Read the model definition and answer for the solid it produces. Units are mm, in the model's axes. Face numbers are marked on the shaded views. Coordinates: 2 decimals unless noted, no trailing zeros. Answer as a JSON object with one key per item and string values. Group by question number.
1) Given pin 1 (1.5 mm diameter, centred on y = -9.5, z = 4, fed in from +X), flat-ended and moving along its own axis, determine where the tip first touches the part or whether it passes through.
2) Consider L1, parallel to X at y = -1.25, z = 0.75; L2, parallel to Y at x = -61, z = 4.75; L3, parallel to X at y = 9.75, z = 5.25. Determine where each line is inside the solid, lowest interval first.
3) Determine the mould class of the marked faces 1, 2 and 3 for opening direction X: released by +X, released by -X, zero draft, split by the parting line, or undercut.
4) Section A-A on z = 3 is taken. Count the separate pieces of the cut face and the enclosed holes in it, and give its area (3 significant figures).
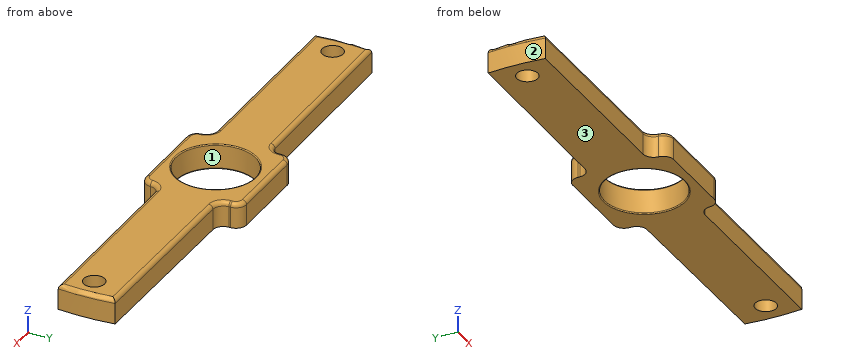
from build123d import *

# Parameters (mm, degrees)
ESQUISSE1_W             = 200
ESQUISSE1_H             = 24
BOSS_EXTRU_1_DEPTH      = 6
ESQUISSE3_R             = 9.5
ENL_V_MAT_EXTRU_1_DEPTH = 6
ESQUISSE4_R             = 114.275088212
ESQUISSE4_R_2           = 60
ENL_V_MAT_EXTRU_2_DEPTH = 6
ESQUISSE5_W             = 52.011744551
ESQUISSE5_H             = 15.54113196
ESQUISSE5_W_2           = 52.011744552
ENL_V_MAT_EXTRU_3_DEPTH = 6
CONG_1_R                = 2.5
CONG_2_R                = 2.5
CONG_3_R                = 1
CONG_4_R                = 0.25
CONG_5_R                = 0.25
ESQUISSE6_R             = 2.5
ENL_V_MAT_EXTRU_4_DEPTH = 68.365782888


with BuildPart() as part:
    # Esquisse1 → Boss.-Extru.1 (new body)
    with BuildSketch(Plane.XY):
        with Locations((-5.765391807, 0)):
            Rectangle(ESQUISSE1_W, ESQUISSE1_H)
    extrude(amount=BOSS_EXTRU_1_DEPTH)

    # Esquisse3 → Enlèv. mat.-Extru.1 (cut)
    with BuildSketch(Plane.XY.offset(6)):
        with Locations((-6.016275927, -0.323603958)):
            Circle(ESQUISSE3_R)
    extrude(amount=-ENL_V_MAT_EXTRU_1_DEPTH, mode=Mode.SUBTRACT)

    # Esquisse4 → Enlèv. mat.-Extru.2 (cut)
    with BuildSketch(Plane.XY.offset(6)):
        with Locations((-6.016275927, -0.323603958)):
            Circle(ESQUISSE4_R)
        with Locations((-6.016275927, -0.323603958)):
            Circle(ESQUISSE4_R_2, mode=Mode.SUBTRACT)
    extrude(amount=-ENL_V_MAT_EXTRU_2_DEPTH, mode=Mode.SUBTRACT)

    # Esquisse5 → Enlèv. mat.-Extru.3 (cut)
    with BuildSketch(Plane.XY.offset(6)):
        Polygon((-69.803207514, 21.817117384), (-17.792224869, 22.098641011), (-17.708105486, 6.557736709), (-69.719088132, 6.276213083), align=None)
        with Locations((-43.676559905, -15.038694091)):
            Rectangle(ESQUISSE5_W, ESQUISSE5_H)
        with Locations((32.145776291, -15.038694091)):
            Rectangle(ESQUISSE5_W_2, ESQUISSE5_H)
        Polygon((58.188304518, 6.276213083), (58.272423901, 21.817117384), (6.261441255, 22.098641011), (6.177321873, 6.557736709), align=None)
    extrude(amount=-ENL_V_MAT_EXTRU_3_DEPTH, mode=Mode.SUBTRACT)

    # Congé1
    cong_1_edges = [part.edges().sort_by_distance(p)[0] for p in [
        (-17.708105486, 6.557736709, 3),
        (6.139904015, -7.268128111, 3),
        (6.177321873, 6.557736709, 3),
        (-17.670687629, -7.268128111, 3),
    ]]
    fillet(cong_1_edges, radius=CONG_1_R)

    # Congé2
    cong_2_edges = [part.edges().sort_by_distance(p)[0] for p in [
        (6.206779607, 12, 3),
        (-17.73756322, 12, 3),
        (-17.670687629, -12, 3),
        (6.139904015, -12, 3),
    ]]
    fillet(cong_2_edges, radius=CONG_2_R)

    # Congé3
    cong_3_edges = [part.edges().sort_by_distance(p)[0] for p in [
        (31.147090613, 6.422581027, 6),
        (-42.891860863, -7.268128111, 6),
        (-17.722797632, 9.272084177, 6),
        (6.913507547, 7.285995677, 6),
        (-18.450972556, -7.953581317, 6),
        (-18.44429116, 7.285995677, 6),
        (-5.765391807, 12, 6),
        (6.192014019, 9.272084177, 6),
        (-5.765391807, -12, 6),
        (6.920188943, -7.953581317, 6),
        (5.366813532, -11.314546795, 6),
        (-16.897597145, -11.314546795, 6),
        (-16.996539353, 11.262976271, 6),
        (5.46575574, 11.262976271, 6),
        (53.983508026, -0.484618209, 6),
        (-66.016056196, -0.485985355, 6),
        (-42.928909262, 6.421222231, 6),
        (31.110193129, -7.268128111, 6),
    ]]
    fillet(cong_3_edges, radius=CONG_3_R)

    # Congé4
    cong_4_edges = [part.edges().sort_by_distance(p)[0] for p in [
        (-15.516275927, -0.323603958, 6),
    ]]
    fillet(cong_4_edges, radius=CONG_4_R)

    # Congé5
    cong_5_edges = [part.edges().sort_by_distance(p)[0] for p in [
        (-15.516275927, -0.323603958, 0),
    ]]
    fillet(cong_5_edges, radius=CONG_5_R)

    # Esquisse6 → Enlèv. mat.-Extru.4 (cut, through all)
    with BuildSketch(Plane.XY.offset(6)):
        with Locations((48.768783674, -1.17977957)):
            Circle(ESQUISSE6_R)
        with Locations((-60.807622013, -0.533809454)):
            Circle(ESQUISSE6_R)
    extrude(amount=-ENL_V_MAT_EXTRU_4_DEPTH, mode=Mode.SUBTRACT)


solid = part.part
Worked answers:
{
 "1": {"pin 1": "stops at x = 6.36"},
 "2": {"L1": "x = -66.01 to -63.2, -58.41 to -15.47, 3.44 to 46.27, 51.27 to 53.98", "L2": "y = -7.27 to -3.03, 1.96 to 6.32", "L3": "x = -17.68 to 6.15"},
 "3": {"face 1": "undercut", "face 2": "released by -X", "face 3": "zero draft"},
 "4": {"separate pieces": "1", "enclosed holes": "3", "area": "1,560 mm²"}
}
